Read the model definition and answer for the solid it produces. Units are mm, in the model's axes. Face numbers are marked on the shaded views. Round coordinates to 2 decimals unless told otherwise and drop trailing zeros. Write each loop counter-clockwise with the first axis right and the second up, starting at its lowest first coordinate (ties: lowest second). Pieces come first, ordered by that corner, then holes. Notation, with made-up numbers: (51.25, 60.5) -> (105.25, 60.5) arc R23 ccw to (105.25, 69.5) -> close; hole circle Ø5 at (66.25, 58.5). An arc over 180 degrees is marked (long way). Return JSON: item names as keys, results as strings. Group by question number.
(1) The mould has two halves that part along X. Classify the marked faces 1, 2 and 3: released by +X, released by -X, zero draft, split by the parting line, or undercut.
(2) Straight lines are drawn through the part: line 1 (X direction, y = -38, z = -5.5); line 2 (Z direction, x = -7, y = -44); line 3 (Y direction, x = 18, z = -8). For each, find the intervals that lie inside material, in ascending order.
(3) A cutting plane is placed at B-B on y = 18.5. Give the vertices of the cut face in (x, z).
(4) A cutting plane is placed at A-A on y = -40. Give the vertices of the cut face in (x, z).
(5) Given pin 1 (2 mm diameter, centred on x = 6, z = 11.5, fed in from -Y); pin 2 (6 mm diameter, centred on x = 4.5, y = 12.5, fed in from +Z); pin 3 (5 mm diameter, centred on y = -18.5, z = -7.5, fed in from -X); pin 4 (8 mm diameter, centred on x = -18.5, y = -20, fed in from +Z), each flat-ended and moving along its own axis, determine where each tip first touches the part or whether it passes through.
(6) A cutting plane is placed at C-C on y = 52. Give the vertices of the cut face in (x, z), then the cut area to 3 significant figures.
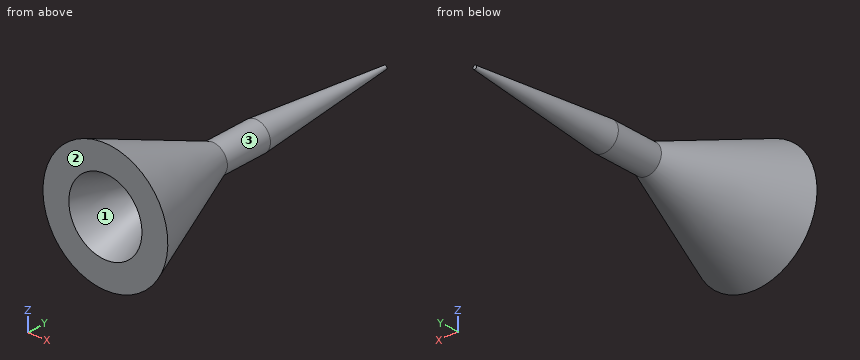
```python
from build123d import *

# Parameters (mm, degrees)
SKETCH1_R           = 6
BOSS_EXTRUDE1_DEPTH = 20
SKETCH2_R           = 26
BOSS_EXTRUDE2_DEPTH = 50
CHAMFER1_SIZE       = 50
CHAMFER1_SIZE_2     = 20
SKETCH3_R           = 6
BOSS_EXTRUDE3_DEPTH = 60
BOSS_EXTRUDE3_TAPER = 5


# Read off the part's stored shape, not the designer's step: Shell1
with BuildPart() as part:
    # Sketch1 → Boss-Extrude1 (new body)
    with BuildSketch(Plane(origin=(0, 0, 0), x_dir=(1, 0, 0), z_dir=(0, 1, 0))):
        with Locations(Location((0, 0, 0), (0, 0, 270))):
            Circle(SKETCH1_R)
    extrude(amount=BOSS_EXTRUDE1_DEPTH)

    # Sketch2 → Boss-Extrude2 (add)
    with BuildSketch(Plane.XZ):
        with Locations(Location((0, 0, 0), (0, 0, 270))):
            Circle(SKETCH2_R)
    extrude(amount=BOSS_EXTRUDE2_DEPTH)

    # Chamfer1
    # the kernel refuses this chamfer: 50, 20 mm, written as the material it takes off along each edge
    with BuildSketch(Plane(origin=(0, 0, 0), x_dir=(0, 0, -1), z_dir=(-1, 0, 0))) as chamfer1_piece_1:
        Polygon((26, CHAMFER1_SIZE), (26 - CHAMFER1_SIZE_2, 0), (26, 0), align=None)
    revolve(axis=Axis((0, 0, 0), (0, -1, 0)), mode=Mode.SUBTRACT)

    # Shell1 outline → Shell1 (revolve, cut)
    with BuildSketch(Plane.XY):
        Polygon((15.229670386, -50), (0, -11.925824036), (0, -50), align=None)
    revolve(axis=Axis((0, 0, 0), (0, 1, 0)), mode=Mode.SUBTRACT)

    # Sketch3 → Boss-Extrude3 (add)
    with BuildSketch(Plane(origin=(0, 20, 0), x_dir=(1, 0, 0), z_dir=(0, 1, 0))):
        with Locations(Location((0, 0, 0), (0, 0, 90))):
            Circle(SKETCH3_R)
    extrude(amount=BOSS_EXTRUDE3_DEPTH, taper=BOSS_EXTRUDE3_TAPER)


solid = part.part
```
Checks:
{
 "1": {"face 1": "undercut", "face 2": "zero draft", "face 3": "split by the parting line"},
 "2": {"line 1": "x = -20.47 to -8.86, 8.86 to 20.47", "line 2": "z = -22.54 to -10.75, 10.75 to 22.54", "line 3": "y = -50 to -34.24"},
 "3": {"outline": "circle Ø12 at (0, 0)"},
 "4": {"outline": "circle Ø44 at (0, 0); hole circle Ø22.46 at (0, 0)"},
 "5": {"pin 1": "stops at y = -46.85", "pin 2": "stops at z = 5.81", "pin 3": "stops at x = -12.89", "pin 4": "passes through"},
 "6": {"outline": "circle Ø6.4 at (0, 0)", "area": "32.2 mm^2"}
}
